Work out the finished part from the listing and answer in its coordinate system (mm). Face numbers are marked on the shaded views. A direction names the side the tool comes from. Give positions to 0.01 mm unless a question says otherwise; leave off trailing zeros. Order: outer loops, then holes, each group sorted by start corner. A loop starts at its lowest first (then second) coordinate and runs counter-clockwise, first axis right, second up.
```python
from build123d import *

# Parameters (mm, degrees)
SKETCH1_W                                       = 30
SKETCH1_H                                       = 30
BOSS_EXTRUDE1_DEPTH                             = 12.7
CSK_FOR_M3_FLAT_HEAD_MACHINE_SCREW1_D           = 3.2
CSK_FOR_M3_FLAT_HEAD_MACHINE_SCREW1_CSINK_D     = 6.3
CSK_FOR_M3_FLAT_HEAD_MACHINE_SCREW1_CSINK_ANGLE = 90


with BuildPart() as part:
    # Sketch1 → Boss-Extrude1 (new body)
    with BuildSketch(Plane.XY):
        Rectangle(SKETCH1_W, SKETCH1_H)
        with BuildLine():
            ThreePointArc((-8.9105463, -5.42101224), (-10.57898776, -5.9105463), (-10.0894537, -7.57898776))
            ThreePointArc((-10.0894537, -7.57898776), (-8.42101224, -7.0894537), (-8.9105463, -5.42101224))
        make_face(mode=Mode.SUBTRACT)
        with BuildLine():
            ThreePointArc((-8.9105463, 7.57898776), (-10.57898776, 7.0894537), (-10.0894537, 5.42101224))
            ThreePointArc((-10.0894537, 5.42101224), (-8.42101224, 5.9105463), (-8.9105463, 7.57898776))
        make_face(mode=Mode.SUBTRACT)
        with BuildLine():
            ThreePointArc((10.0894537, 7.57898776), (8.42101224, 7.0894537), (8.9105463, 5.42101224))
            ThreePointArc((8.9105463, 5.42101224), (10.57898776, 5.9105463), (10.0894537, 7.57898776))
        make_face(mode=Mode.SUBTRACT)
        with BuildLine():
            ThreePointArc((10.0894537, -5.42101224), (8.42101224, -5.9105463), (8.9105463, -7.57898776))
            ThreePointArc((8.9105463, -7.57898776), (10.57898776, -7.0894537), (10.0894537, -5.42101224))
        make_face(mode=Mode.SUBTRACT)
        with BuildLine():
            add(Edge.make_bspline(
                [(-1.342391508, -9.257231173), (-1.831415943, -8.990075907), (-2.180549698, -8.556474598), (-2.530193945, -8.122239293), (-2.686738964, -7.588310687), (-2.84359347, -7.053326516), (-2.783896578, -6.500133621), (-2.724081666, -5.945847074), (-2.457231173, -5.457608492), (-2.189853123, -4.968404672), (-1.756474598, -4.619450302), (-1.322239293, -4.269806055), (-0.788310687, -4.113261036), (-0.253326516, -3.95640653), (0.299866379, -4.016103422), (0.853868841, -4.075887677), (1.342391508, -4.342768827)],
                knots=[0, 0, 0, 0.125, 0.125, 0.25, 0.25, 0.375, 0.375, 0.5, 0.5, 0.625, 0.625, 0.75, 0.75, 0.875, 0.875, 1, 1, 1], degree=2))
            add(Edge.make_bspline(
                [(1.342391508, -4.342768827), (1.831415943, -4.609924093), (2.180549698, -5.043525402), (2.530193945, -5.477760707), (2.686738964, -6.011689313), (2.84359347, -6.546673484), (2.783896578, -7.099866379), (2.724081666, -7.654152926), (2.457231173, -8.142391508), (2.189853123, -8.631595328), (1.756474598, -8.980549698), (1.322239293, -9.330193945), (0.788310687, -9.486738964), (0.253326516, -9.64359347), (-0.299866379, -9.583896578), (-0.853868841, -9.524112323), (-1.342391508, -9.257231173)],
                knots=[0, 0, 0, 0.125, 0.125, 0.25, 0.25, 0.375, 0.375, 0.5, 0.5, 0.625, 0.625, 0.75, 0.75, 0.875, 0.875, 1, 1, 1], degree=2))
        make_face(mode=Mode.SUBTRACT)
        with BuildLine():
            add(Edge.make_bspline(
                [(1.342391508, 9.257231173), (1.831415943, 8.990075907), (2.180549698, 8.556474598), (2.530193945, 8.122239293), (2.686738964, 7.588310687), (2.84359347, 7.053326516), (2.783896578, 6.500133621), (2.724081666, 5.945847074), (2.457231173, 5.457608492), (2.189853123, 4.968404672), (1.756474598, 4.619450302), (1.322239293, 4.269806055), (0.788310687, 4.113261036), (0.253326516, 3.95640653), (-0.299866379, 4.016103422), (-0.853868841, 4.075887677), (-1.342391508, 4.342768827)],
                knots=[0, 0, 0, 0.125, 0.125, 0.25, 0.25, 0.375, 0.375, 0.5, 0.5, 0.625, 0.625, 0.75, 0.75, 0.875, 0.875, 1, 1, 1], degree=2))
            add(Edge.make_bspline(
                [(-1.342391508, 4.342768827), (-1.831415943, 4.609924093), (-2.180549698, 5.043525402), (-2.530193945, 5.477760707), (-2.686738964, 6.011689313), (-2.84359347, 6.546673484), (-2.783896578, 7.099866379), (-2.724081666, 7.654152926), (-2.457231173, 8.142391508), (-2.189853123, 8.631595328), (-1.756474598, 8.980549698), (-1.322239293, 9.330193945), (-0.788310687, 9.486738964), (-0.253326516, 9.64359347), (0.299866379, 9.583896578), (0.853868841, 9.524112323), (1.342391508, 9.257231173)],
                knots=[0, 0, 0, 0.125, 0.125, 0.25, 0.25, 0.375, 0.375, 0.5, 0.5, 0.625, 0.625, 0.75, 0.75, 0.875, 0.875, 1, 1, 1], degree=2))
        make_face(mode=Mode.SUBTRACT)
    extrude(amount=BOSS_EXTRUDE1_DEPTH)

    # CSK for M3 Flat Head Machine Screw1 (through all)
    with Locations(Plane.XY.offset(12.7)):
        with Locations((-9.5, -6.5), (-9.5, 6.5), (9.5, 6.5), (9.5, -6.5)):
            CounterSinkHole(CSK_FOR_M3_FLAT_HEAD_MACHINE_SCREW1_D / 2, CSK_FOR_M3_FLAT_HEAD_MACHINE_SCREW1_CSINK_D / 2, counter_sink_angle=CSK_FOR_M3_FLAT_HEAD_MACHINE_SCREW1_CSINK_ANGLE)

    # Sketch10 → 1/8 NPT Tapped Hole1 (revolve, cut)
    with BuildSketch(Plane(origin=(-0.014274842, -6.826129923, 12.7), x_dir=(0, -1, 0), z_dir=(1, 0, 0))):
        Polygon((0, 0), (0, 12.134668714), (4.2164, 9.6012), (4.2164, 6.92), (4.537398933, 6.92), (4.744593, 0), align=None)
    f_1_8_npt_tapped_hole1 = revolve(axis=Axis((-0.014274842, -6.826129923, 19.05), (0, 0, -1)), mode=Mode.SUBTRACT)

    # Mirror1: 1/8 NPT Tapped Hole1 across plane
    add(f_1_8_npt_tapped_hole1.mirror(Plane.ZX), mode=Mode.SUBTRACT)


solid = part.part
```
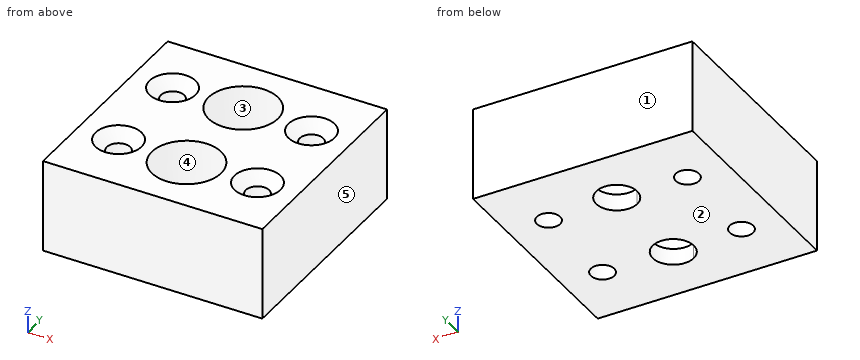
1. The part is cut by section A-A (x = -9.5). Write down the section's boundary in (y, z), then the cut area to 3 significant figures.
Findings below:
outline: (-15, 0) - (-8.1, 0) - (-8.1, 11.15) - (-9.65, 12.7) - (-15, 12.7) - close; (-4.9, 0) - (4.9, 0) - (4.9, 11.15) - (3.35, 12.7) - (-3.35, 12.7) - (-4.9, 11.15) - close; (8.1, 0) - (15, 0) - (15, 12.7) - (9.65, 12.7) - (8.1, 11.15) - close
area: 295 mm2
2. The part is cut by section D-D (z = 8.5). Write down the section's boundary in (x, y), then the cut area to 3 significant figures.
Findings below:
outline: (-15, -15) - (15, -15) - (15, 15) - (-15, 15) - close; hole circle Ø3.2 at (-9.5, -6.5); hole circle Ø3.2 at (-9.5, 6.5); hole circle Ø9.24 at (-0.01, -6.83); hole circle Ø9.24 at (-0.01, 6.83); hole circle Ø3.2 at (9.5, -6.5); hole circle Ø3.2 at (9.5, 6.5)
area: 734 mm2
3. The mould has two halves that part along Y. Classify the marked faces 1, 2 and 3: pulls with the +Y half, pulls with the -Y half, needs draft (parallel to the pull), parting line crosses it, or undercut.
Findings below:
face 1: pulls with the +Y half
face 2: needs draft
face 3: undercut
4. Which of the six approach directions +Z, -Z, +X, -X, +Y, -Y give full straight-line access (tool end or side, diameter ignored) to the marked faces 4 and 5?
Findings below:
face 4: +Z
face 5: +Z, -Z, +X, +Y, -Y
5. The part is cut by section B-B (z = 1.25). State how many separate pieces and enclosed holes the cut face has, then the cut area to 3 significant figures.
Findings below:
separate pieces: 1
enclosed holes: 6
area: 819 mm2
6. Given P1, Ø5, axis at x = -0.01, y = 6.83, coming from the +Z side; P2, Ø5, axis at x = 9.5, y = -6.5, coming from the +Z side, each flat-ended and moving along its own axis, determine where each tip first touches the part or whether it passes through.
Findings below:
P1: passes through
P2: stops at z = 12.05
7. Straight lines are drawn through the part: probe 1 along Y at (x, z) = (9.5, 6.5); probe 2 along Y at (x, z) = (-1.5, 2.5); probe 3 along X at (y, z) = (6.5, 5). For each, find the intervals that lie inside material, in ascending order.
Findings below:
probe 1: y = -15 to -8.1, -4.9 to 4.9, 8.1 to 15
probe 2: y = -15 to -9.68, -3.97 to 3.97, 9.68 to 15
probe 3: x = -15 to -11.1, -7.9 to -4.22, 4.19 to 7.9, 11.1 to 15
